Can you work these out from the model? Positions are in its coordinate system, mm. A direction names the side the tool comes from. Coordinates: 2 decimals unless noted, no trailing zeros. Loops run counter-clockwise (first coordinate to the right, second up) from the corner with the lowest first, then second, coordinate; pieces in that order, holes last.
```python
from build123d import *

# Parameters (mm, degrees)
SKETCH1_R           = 2.9
BOSS_EXTRUDE1_DEPTH = 45.2
SKETCH2_R           = 3.7
BOSS_EXTRUDE2_DEPTH = 1
FILLET2_R           = 1
BOSS_EXTRUDE3_DEPTH = 1.4
SKETCH4_R           = 1
SKETCH5_R           = 2.9


with BuildPart() as part:
    # Sketch1 → Boss-Extrude1 (new body)
    with BuildSketch(Plane(origin=(0, 0, 0), x_dir=(1, 0, 0), z_dir=(0, 1, 0))):
        with Locations(Location((0, 0, 0), (0, 0, 270))):
            Circle(SKETCH1_R)
    extrude(amount=BOSS_EXTRUDE1_DEPTH)

    # Sketch2 → Boss-Extrude2 (add)
    with BuildSketch(Plane.XZ):
        with Locations(Location((0, 0, 0), (0, 0, 270))):
            Circle(SKETCH2_R)
    extrude(amount=BOSS_EXTRUDE2_DEPTH)

    # Fillet2
    # the kernel refuses this fillet: 1 mm, written as the material it takes off along each edge
    with BuildSketch(Plane(origin=(0, 0, 0), x_dir=(0, 0, -1), z_dir=(-1, 0, 0))) as fillet2_piece_1:
        with BuildLine():
            CenterArc((2.7, 0.979795897), FILLET2_R, 281.536959033, 78.463040967)
            Line((2.9, 0), (2.904, -0.019595918))
            ThreePointArc((2.904, -0.019595918), (3.3, -0.02), (3.7, -0.02))
            Line((3.7, -0.02), (3.72, 0))
            Line((3.72, 0), (3.72, 0.979795897))
            Line((3.72, 0.979795897), (3.7, 0.979795897))
        make_face()
    revolve(axis=Axis((0, 0, 0), (0, -1, 0)), mode=Mode.SUBTRACT)

    # Sketch3 → Boss-Extrude3 (add)
    with BuildSketch(Plane(origin=(0, 17.2, 0), x_dir=(1, 0, 0), z_dir=(0, 1, 0))):
        with BuildLine():
            ThreePointArc((0, 10.15), (-10.15, 0), (0, -10.15))
            Line((0, -10.15), (0, -8))
            ThreePointArc((0, -8), (-1.5, -6.5), (0, -5))
            Line((0, -5), (0, 5))
            ThreePointArc((0, 5), (-1.5, 6.5), (0, 8))
            Line((0, 8), (0, 10.15))
        make_face()
        with BuildLine():
            Line((0, -8), (0, -10.15))
            ThreePointArc((0, -10.15), (7.177133829, -7.177133829), (10.15, 0))
            ThreePointArc((10.15, 0), (7.177133829, 7.177133829), (0, 10.15))
            Line((0, 10.15), (0, 8))
            ThreePointArc((0, 8), (1.060660172, 7.560660172), (1.5, 6.5))
            ThreePointArc((1.5, 6.5), (1.060660172, 5.439339828), (0, 5))
            Line((0, 5), (0, -5))
            ThreePointArc((0, -5), (1.060660172, -5.439339828), (1.5, -6.5))
            ThreePointArc((1.5, -6.5), (1.060660172, -7.560660172), (0, -8))
        make_face()
    extrude(amount=-BOSS_EXTRUDE3_DEPTH)

    # Sketch4 → Loft1 section 0
    with BuildSketch(Plane(origin=(0, 51.7, 0), x_dir=(1, 0, 0), z_dir=(0, 1, 0))):
        Circle(SKETCH4_R)
    # Sketch5 → Loft1 section 1
    with BuildSketch(Plane(origin=(0, 45.2, 0), x_dir=(1, 0, 0), z_dir=(0, 1, 0))):
        Circle(SKETCH5_R)
    loft()


solid = part.part
```
Item 1: On a 3-axis mill with a long thin cutter (end or side, diameter ignored), from which of +Z, -Z, +X, -X, +Y, -Y can I reach the whole of each face in a straight line? I mean faces 1 (the face through (0, -1, 0)), 2 (the face through (0.1, 31, -2.9)), 3 (the face through (0.1, 7.8, -2.9)). Say none if no direction works.
Results are:
face 1: +Z, -Z, +X, -X, -Y
face 2: +Y
face 3: none
Item 2: Suppose I cut it at B-B, the plane x = -6.25. Please give me the cut outline in (y, z).
Results are:
outline: (15.8, -8) - (17.2, -8) - (17.2, 8) - (15.8, 8) - close
Item 3: Suppose I cut it at C-C, the plane y = 47.5. Please give me the cut outline in (x, z).
Results are:
outline: circle Ø4.46 at (0, 0)
Item 4: Suppose I cut it at A-A, the plane y = 27. Please give me the cut outline in (x, z), plus the area to 3 significant figures.
Results are:
outline: circle Ø5.8 at (0, 0)
area: 26.4 mm2
Item 5: I'm going to push flat-ended pins straight in: P1, Ø3, axis at x = 2, y = 39, coming from the +Z side; P2, Ø5, axis at y = 28.5, z = -1, coming from the -X side; P3, Ø3, axis at x = 3, y = 14, coming from the -Z side; P4, Ø6, axis at x = -3, z = 0.5, coming from the +Y side. Where does each tip first touch, or does it pass through?
Results are:
P1: stops at z = 2.86
P2: stops at x = -2.9
P3: stops at z = -2.48
P4: stops at y = 51.7
Item 6: I need wall thicknesses on line 1 along Y through (x, z) = (4.5, -8.5); line 2 along X through (y, z) = (29, -1.25); line 3 along Z through (x, y) = (-1, 30.5). Which ranges of each line are inside material? Lowest first, please.
Results are:
line 1: y = 15.8 to 17.2
line 2: x = -2.62 to 2.62
line 3: z = -2.72 to 2.72
